```python
from build123d import *

# Parameters (mm, degrees)
SKETCH1_R                = 7.9375
BOSS_EXTRUDE1_DEPTH      = 29.972
W_0_386_DIAMETER_HOLE1_D = 9.8044
CHAMFER1_SIZE            = 0.4


with BuildPart() as part:
    # Sketch1 → Boss-Extrude1 (new body)
    with BuildSketch(Plane(origin=(0, 0, 0), x_dir=(1, 0, 0), z_dir=(0, 1, 0))):
        with Locations(Location((0, 0, 0), (0, 0, 90))):
            Circle(SKETCH1_R)
    extrude(amount=BOSS_EXTRUDE1_DEPTH)

    # W (0.386) Diameter Hole1 (through all)
    with Locations(Plane(origin=(0, 29.972, 0), x_dir=(1, 0, 0), z_dir=(0, 1, 0))):
        with Locations((0, 0)):
            Hole(W_0_386_DIAMETER_HOLE1_D / 2)

    # Chamfer1
    chamfer1_edges = [part.edges().sort_by_distance(p)[0] for p in [
        (4.9022, 29.972, 0),
        (4.9022, 0, 0),
    ]]
    chamfer(chamfer1_edges, length=CHAMFER1_SIZE)


solid = part.part
```
Geometry check sheet. Reference: the model listing, model coordinates, mm. Coordinates: 2 decimals unless noted, no trailing zeros. Order: outer loops, then holes, each group sorted by start corner. A loop starts at its lowest first (then second) coordinate and runs counter-clockwise, first axis right, second up.
Q1. Sectioned sample at C-C on z = 6.25. Record the cut outline in (x, y).
Reply:
outline: (-4.89, 0) - (4.89, 0) - (4.89, 29.97) - (-4.89, 29.97) - close
Q2. Sectioned sample at B-B on y = 2.5. Record the cut outline in (x, z) (1 decimal), and give its area (3 significant figures).
Reply:
outline: circle Ø15.9 at (0, 0); hole circle Ø9.8 at (0, 0)
area: 122 mm2
Q3. Depth check by flat-ended pin: pin 1 Ø2 at (y, z) = (18, -5.5) entering from +X; pin 2 Ø2 at (y, z) = (26.5, 3.5) entering from -X; pin 3 Ø2 at (y, z) = (19.5, -0.5) entering from -X; pin 4 Ø1 at (x, y) = (-3.5, 15.5) entering from +Z. Enter the tip coordinate at first touch or a pass-through.
Reply:
pin 1: stops at x = 6.54
pin 2: stops at x = -7.53
pin 3: stops at x = -7.94
pin 4: stops at z = 7.35
Q4. Sectioned sample at A-A on z = 0. Record the cut outline in (x, y), and give its area (3 significant figures).
Reply:
outline: (-7.94, 0) - (-5.3, 0) - (-4.9, 0.4) - (-4.9, 29.57) - (-5.3, 29.97) - (-7.94, 29.97) - close; (4.9, 0.4) - (5.3, 0) - (7.94, 0) - (7.94, 29.97) - (5.3, 29.97) - (4.9, 29.57) - close
area: 182 mm2
Q5. Thickness scan on probe 1 along X at (y, z) = (19.25, 0); probe 2 along X at (y, z) = (23, 4); probe 3 along Z at (x, y) = (-2.75, 8.5). Record the ranges inside material, lowest first.
Reply:
probe 1: x = -7.94 to -4.9, 4.9 to 7.94
probe 2: x = -6.86 to -2.83, 2.83 to 6.86
probe 3: z = -7.45 to -4.06, 4.06 to 7.45
Q6. Draft check along Z on faces 1 (the face through (5.2, 29.972, -1.7)), 2 (the face through (-4.676, 14.782, -1.472)), 3 (the face through (7.75, 14.78, 1.72)). Enter one of: released by +Z, released by -Z, zero draft, split by the parting line, or undercut.
Reply:
face 1: zero draft
face 2: undercut
face 3: split by the parting line
